from build123d import *

# Parameters (mm, degrees)
SKETCH1_R           = 9.144
BOSS_EXTRUDE1_DEPTH = 70.104


with BuildPart() as part:
    # Sketch1 → Boss-Extrude1 (new body)
    with BuildSketch(Plane.XY):
        with BuildLine():
            Line((0, 20.32), (-0.635, 20.32))
            Line((-0.635, 20.32), (-0.635, 21.580659744))
            ThreePointArc((-0.635, 21.580659744), (-19.006899569, 10.973638583), (-19.006899569, -10.240403741))
            Line((-19.006899569, -10.240403741), (-17.915136205, -9.610073869))
            Line((-17.915136205, -9.610073869), (-17.597636205, -10.16))
            Line((-17.597636205, -10.16), (-17.280136205, -10.709926131))
            Line((-17.280136205, -10.709926131), (-18.371899569, -11.340256004))
            ThreePointArc((-18.371899569, -11.340256004), (0, -21.947277165), (18.371899569, -11.340256004))
            Line((18.371899569, -11.340256004), (17.280136205, -10.709926131))
            Line((17.280136205, -10.709926131), (17.597636205, -10.16))
            Line((17.597636205, -10.16), (17.915136205, -9.610073869))
            Line((17.915136205, -9.610073869), (19.025544668, -10.205721439))
            ThreePointArc((19.025544668, -10.205721439), (18.996550601, 10.990773387), (0.635, 21.580659744))
            Line((0.635, 21.580659744), (0.635, 20.32))
            Line((0.635, 20.32), (0, 20.32))
        make_face()
        with Locations((0.118855304, -11.557)):
            Circle(SKETCH1_R, mode=Mode.SUBTRACT)
        with Locations((9.955579479, 5.869470694)):
            Circle(SKETCH1_R, mode=Mode.SUBTRACT)
        with Locations((-10.060900468, 5.687049391)):
            Circle(SKETCH1_R, mode=Mode.SUBTRACT)
    extrude(amount=BOSS_EXTRUDE1_DEPTH)


solid = part.part
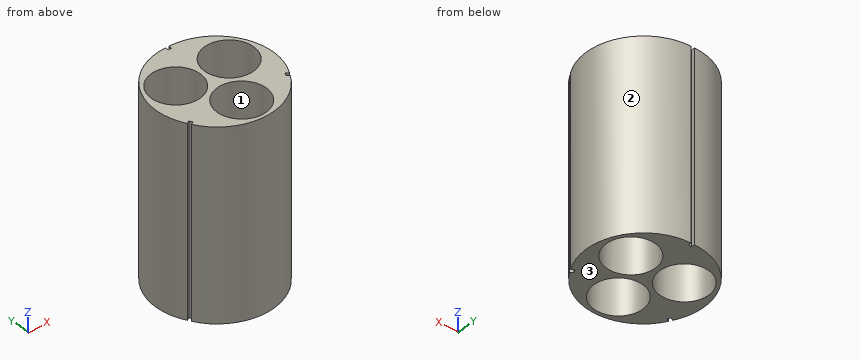
Could you check a few things on this model? Use its own coordinates, in mm. Face numbers are marked on the shaded views. Round coordinates to 2 decimals unless told otherwise and drop trailing zeros. Write each loop counter-clockwise with the first axis right and the second up, starting at its lowest first coordinate (ties: lowest second). Pieces come first, ordered by that corner, then holes. Notation, with made-up numbers: (-29.75, 89.25) - (-16.75, 89.25) arc R25 ccw to (-16.75, 116.25) - close; hole circle Ø10 at (-17.5, -17.75). An arc over 180 degrees is marked (long way). Use a Markdown table: item, result.
Q1. Thinking about a two-plate mould opening in Y: for the marked faces 1, 2 and 3, which applies, released by +Y, released by -Y, zero draft, split by the parting line, or undercut?
Output values:
| item | result |
|---|---|
| face 1 | undercut |
| face 2 | split by the parting line |
| face 3 | zero draft |
Q2. I want a section at C-C (y = 2.5). List the corners of the cut face in (x, z) for me, plus the area to 3 significant figures.
Output values:
| item | result |
|---|---|
| outline | (-21.74, 0) - (-18.63, 0) - (-18.63, 70.1) - (-21.74, 70.1) - close; (-1.49, 0) - (1.46, 0) - (1.46, 70.1) - (-1.49, 70.1) - close; (18.46, 0) - (21.74, 0) - (21.74, 70.1) - (18.46, 70.1) - close |
| area | 655 mm2 |
Q3. I want a section at B-B (x = 5.5). List the corners of the cut face in (y, z) for me, plus the area to 3 significant figures.
Output values:
| item | result |
|---|---|
| outline | (-21.22, 0) - (-18.95, 0) - (-18.95, 70.1) - (-21.22, 70.1) - close; (-4.16, 0) - (-2.12, 0) - (-2.12, 70.1) - (-4.16, 70.1) - close; (13.85, 0) - (21.02, 0) - (21.02, 70.1) - (13.85, 70.1) - close |
| area | 805 mm2 |
Q4. I want a section at A-A (y = -6). List the corners of the cut face in (x, z) for me, plus the area to 3 significant figures.
Output values:
| item | result |
|---|---|
| outline | (-20.87, 0) - (-7.14, 0) - (-7.14, 70.1) - (-20.87, 70.1) - close; (7.38, 0) - (20.87, 0) - (20.87, 70.1) - (7.38, 70.1) - close |
| area | 1,910 mm2 |
Q5. For pin 1 (3 mm diameter, centred on y = -5.5, z = 45.5, fed in from -X); pin 2 (1.5 mm diameter, centred on x = -10.5, z = 25, fed in from +Y); pin 3 (3 mm diameter, centred on x = -5, z = 49, fed in from +Y); pin 4 (21 mm diameter, centred on x = 9.96, y = 5.87, fed in from -Z), each with a flat end and sliding along its axis, tell me the tip position at first contact or that it passes through.
Output values:
| item | result |
|---|---|
| pin 1 | x = -21.39 |
| pin 2 | y = 19.52 |
| pin 3 | y = 21.39 |
| pin 4 | z = 0 |
Q6. Please list where these lines run through material, in increasing order: L1, parallel to X at y = -1, z = 56; L2, parallel to X at y = 7.5, z = 46.5; L3, parallel to Y at x = -4, z = 18.
Output values:
| item | result |
|---|---|
| L1 | -21.8 to -16.3, -3.82 to 3.92, 15.99 to 21.8 |
| L2 | -20.61 to -19.02, -1.1 to 0.96, 18.95 to 20.61 |
| L3 | -21.57 to -19.72, -3.39 to -1.16, 12.53 to 21.31 |
Q7. I want a section at D-D (z = 25.5). List the corners of the cut face in (x, y) for me (3 decimals).
Output values:
| item | result |
|---|---|
| outline | (-19.007, -10.24) - (-17.915, -9.61) - (-17.28, -10.71) - (-18.372, -11.34) arc R21.214 ccw to (18.372, -11.34) - (17.28, -10.71) - (17.915, -9.61) - (19.026, -10.206) arc R21.213 ccw to (0.635, 21.581) - (0.635, 20.32) - (-0.635, 20.32) - (-0.635, 21.581) arc R21.214 ccw to start; hole circle Ø18.288 at (-10.061, 5.687); hole circle Ø18.288 at (0.119, -11.557); hole circle Ø18.288 at (9.956, 5.869) |
